Verification items for the finished model (mm, model axes). A direction names the side the tool comes from. Coordinates: 2 decimals unless noted, no trailing zeros. Write each loop counter-clockwise with the first axis right and the second up, starting at its lowest first coordinate (ties: lowest second). Pieces come first, ordered by that corner, then holes. Notation, with made-up numbers: (86.5, 43) - (115.5, 43) arc R33 cw to (115.5, 72) - close; hole circle Ø6 at (74, 3.25). An arc over 180 degrees is marked (long way). Use one line per item in the form item = value. Start each with the question number.
(1) Sectioned sample at B-B (x = 43.05). Record the cut outline in (y, z).
(2) Gauge pin test, flat ends, axial feed: pin 1 Ø1 at (x, y) = (34, 7) entering from +Z; pin 2 Ø0.8 at (y, z) = (8, -11.5) entering from -X; pin 3 Ø3 at (y, z) = (5, 3) entering from +X (3 decimals). Record the tip position at first contact, or that the pin passes through.
(3) Tool access check on faces 1 (the flat face through (25.95, 4, -5)), 2 (the flat face through (36, 5, -12)), 3 (the flat face through (34.05, 10, -6)), 4 (the flat face through (13, 1.5, -5)), 5 (the flat face through (34.05, 4, -6)). Record the directions out of +Z, -Z, +X, -X, +Y, -Y that give a thin tool (end or side, any length) a straight path to the whole face; none if there is none.
(4) Sectioned sample at D-D (x = 0.5). Record the cut outline in (y, z).
(5) Sectioned sample at A-A (y = 3.5). Count the separate pieces of the cut face and the enclosed holes in it, and give its area (3 significant figures).
(6) Sectioned sample at C-C (y = 9.5). Record the cut outline in (x, z) (3 decimals), and give its area (3 significant figures).
(7) Material ranges on line 1 (Z direction, x = 12.5, y = 10.5); line 2 (Z direction, x = 12, y = 0.8); line 3 (X direction, y = 3.6, z = -0.5), recorded low to high. Write a range as [from, to].
(8) Mould release check, pull along Z, two halves, no side actions. Record for faces 6 (the flat face through (36, 5, 1)), 7 (the flat face through (27.18, 0.49, -9.73)), 8 (the flat face through (21.025, 7, -14)): released by +Z, released by -Z, zero draft, split by the parting line, or undercut.
from build123d import *
from build123d.topology import SkipClean

# Parameters (mm, degrees)
ESQUISSE2_W                 = 36.05
ESQUISSE2_H                 = 13
ESQUISSE2_W_2               = 34.05
ESQUISSE2_H_2               = 11
BOSS_EXTRU_1_DEPTH          = 12
ESQUISSE3_W                 = 13
ESQUISSE3_H                 = 1
BOSS_EXTRU_2_DEPTH          = 36.05
ESQUISSE4_R                 = 2.6
ENL_V_MAT_EXTRU_1_DEPTH     = 12
ESQUISSE6_W                 = 3.9
ESQUISSE6_H                 = 1.5
ESQUISSE6_H_2               = 5
ESQUISSE6_H_3               = 7
BOSS_EXTRU_3_DEPTH          = 13
ENL_V_START                 = -6
ENL_V_MAT_EXTRU_2_OUTLINE_R = 0.8
ENL_V_MAT_EXTRU_2_DEPTH     = 6
ESQUISSE8_W                 = 13
ESQUISSE8_H                 = 6.5
ENL_V_MAT_EXTRU_3_DEPTH     = 40.261972696
ESQUISSE9_W                 = 8.1
ESQUISSE9_H                 = 11
BOSS_EXTRU_5_DEPTH          = 1.4
ESQUISSE11_R                = 2.5
ENL_V_MAT_EXTRU_4_DEPTH     = 38.987662471
CONG_2_R                    = 2
ESQUISSE10_W                = 8.1
ESQUISSE10_H                = 11
ENL_V_MAT_EXTRU_5_DEPTH     = 0.8
BOSS_EXTRU_6_DEPTH          = 2.6
ESQUISSE14_R                = 0.5
ENL_V_MAT_EXTRU_7_DEPTH     = 39.645860063
ESQUISSE15_R                = 0.8
ENL_V_MAT_EXTRU_8_DEPTH     = 38.702818197
ESQUISSE16_W                = 3.3
ESQUISSE16_H                = 13
ENL_V_MAT_EXTRU_9_DEPTH     = 1
CHANFREIN1_SIZE             = 0.5
ESQUISSE18_W                = 15
ESQUISSE18_H                = 13
ESQUISSE18_R                = 0.75
BOSS_EXTRU_9_DEPTH          = 5.5
ESQUISSE19_R                = 1.5
BOSS_EXTRU_10_DEPTH         = 12
ENL_V_MAT_EXTRU_10_DEPTH    = 39.061800076
ESQUISSE23_R                = 3.6
ESQUISSE23_R_2              = 2.6
BOSS_EXTRU_11_DEPTH         = 2


# Read off the part's stored shape, not the designer's step: Enlèv. mat.-Extru.2
with BuildPart() as part:
    # Esquisse2 → Boss.-Extru.1 (new body)
    # profile 1 of 3: a face of its own
    with BuildSketch(Plane(origin=(0, 0, 0), x_dir=(1, 0, 0), z_dir=(0, 1, 0))):
        with Locations((17.025, 5.5)):
            Rectangle(ESQUISSE2_W, ESQUISSE2_H)
        with Locations((17.025, 5.5)):
            Rectangle(ESQUISSE2_W_2, ESQUISSE2_H_2, mode=Mode.SUBTRACT)
    # profile 2 of 3: a face of its own
    with BuildSketch(Plane(origin=(0, 0, 0), x_dir=(1, 0, 0), z_dir=(0, 1, 0))):
        Polygon((0, 0), (2.560660172, 0), (0, 2.560660172), align=None)
    # profile 3 of 3: a face of its own
    with BuildSketch(Plane(origin=(0, 0, 0), x_dir=(1, 0, 0), z_dir=(0, 1, 0))):
        Polygon((0, 11), (0, 8.439339828), (2.560660172, 11), align=None)
    extrude(amount=BOSS_EXTRU_1_DEPTH)

    # Esquisse3 → Boss.-Extru.2 (add)
    with BuildSketch(Plane.ZY.offset(1)):
        with Locations((-5.5, 0.5)):
            Rectangle(ESQUISSE3_W, ESQUISSE3_H)
    extrude(amount=-BOSS_EXTRU_2_DEPTH)

    # Esquisse4 → Enlèv. mat.-Extru.1 (cut)
    with BuildSketch(Plane.XZ):
        with Locations(Location((6, -5.5, 0), (0, 0, 270))):
            Circle(ESQUISSE4_R)
        Polygon((34.05, 0), (28.45, 0), (25.95, -2.5), (25.95, -8.5), (28.45, -11), (34.05, -11), align=None)
    extrude(amount=-ENL_V_MAT_EXTRU_1_DEPTH, mode=Mode.SUBTRACT)

    # Esquisse6 → Boss.-Extru.3 (add)
    with BuildSketch(Plane.XY.offset(1)):
        with Locations((12, 0.75)):
            Rectangle(ESQUISSE6_W, ESQUISSE6_H)
        with Locations((18, 2.5)):
            Rectangle(ESQUISSE6_W, ESQUISSE6_H_2)
        with Locations((24, 3.5)):
            Rectangle(ESQUISSE6_W, ESQUISSE6_H_3)
    extrude(amount=-BOSS_EXTRU_3_DEPTH)

    # Enlèv. mat.-Extru.2 outline → Enlèv. mat.-Extru.2 (cut)
    with BuildSketch(Plane(origin=(0, 7, 0), x_dir=(1, 0, 0), z_dir=(0, 1, 0)).offset(ENL_V_START)):
        with BuildLine():
            Line((24, 7.45), (24, 11))
            Line((24, 11), (22.05, 11))
            Line((22.05, 11), (22.05, 5.5))
            ThreePointArc((22.05, 5.5), (22.621141777, 6.878858223), (24, 7.45))
        make_face()
        with BuildLine():
            Line((19.95, 5.5), (19.95, 11))
            Line((19.95, 11), (16.05, 11))
            Line((16.05, 11), (16.05, 5.5))
            ThreePointArc((16.05, 5.5), (18, 7.45), (19.95, 5.5))
        make_face()
        with BuildLine():
            ThreePointArc((24, 3.55), (22.621141777, 4.121141777), (22.05, 5.5))
            Line((22.05, 5.5), (22.05, 0))
            Line((22.05, 0), (24, 0))
            Line((24, 0), (24, 3.55))
        make_face()
        with BuildLine():
            Line((19.95, 0), (19.95, 5.5))
            ThreePointArc((19.95, 5.5), (18, 3.55), (16.05, 5.5))
            Line((16.05, 5.5), (16.05, 0))
            Line((16.05, 0), (19.95, 0))
        make_face()
        with BuildLine():
            Line((13.95, 5.5), (13.95, 11))
            Line((13.95, 11), (10.05, 11))
            Line((10.05, 11), (10.05, 5.5))
            ThreePointArc((10.05, 5.5), (12, 7.45), (13.95, 5.5))
        make_face()
        with BuildLine():
            Line((13.95, 0), (13.95, 5.5))
            ThreePointArc((13.95, 5.5), (12, 3.55), (10.05, 5.5))
            Line((10.05, 5.5), (10.05, 0))
            Line((10.05, 0), (13.95, 0))
        make_face()
        with Locations((24, 5.5)):
            Circle(ENL_V_MAT_EXTRU_2_OUTLINE_R)
        with Locations((18, 5.5)):
            Circle(ENL_V_MAT_EXTRU_2_OUTLINE_R)
        with Locations((12, 5.5)):
            Circle(ENL_V_MAT_EXTRU_2_OUTLINE_R)
    extrude(amount=ENL_V_MAT_EXTRU_2_DEPTH, mode=Mode.SUBTRACT)

    # Esquisse8 → Enlèv. mat.-Extru.3 (cut, through all)
    with BuildSketch(Plane(origin=(0, 0, -12), x_dir=(-1, 0, 0), z_dir=(0, 0, -1))):
        with Locations((-5.5, 8.75)):
            Rectangle(ESQUISSE8_W, ESQUISSE8_H)
    extrude(amount=-ENL_V_MAT_EXTRU_3_DEPTH, mode=Mode.SUBTRACT)

    # Esquisse9 → Boss.-Extru.5 (add)
    with BuildSketch(Plane(origin=(0, 7, 0), x_dir=(1, 0, 0), z_dir=(0, 1, 0))):
        with Locations((30, 5.5)):
            Rectangle(ESQUISSE9_W, ESQUISSE9_H)
        with BuildLine():
            Line((24, 0), (25.95, 0))
            Line((25.95, 0), (25.95, 11))
            Line((25.95, 11), (24, 11))
            Line((24, 11), (24, 7.45))
            Line((24, 7.45), (24, 7.25))
            ThreePointArc((24, 7.25), (25.237436867, 6.737436867), (25.75, 5.5))
            ThreePointArc((25.75, 5.5), (25.237436867, 4.262563133), (24, 3.75))
            Line((24, 3.75), (24, 3.55))
            Line((24, 3.55), (24, 0))
        make_face()
    extrude(amount=BOSS_EXTRU_5_DEPTH)

    # Esquisse11 → Enlèv. mat.-Extru.4 (cut, through all)
    with BuildSketch(Plane(origin=(0, 8.4, 0), x_dir=(1, 0, 0), z_dir=(0, 1, 0))):
        with Locations(Location((30, 5.5, 0), (0, 0, 180))):
            Circle(ESQUISSE11_R)
    extrude(amount=-ENL_V_MAT_EXTRU_4_DEPTH, mode=Mode.SUBTRACT)

    # Congé2
    # the kernel refuses this fillet: 2 mm, written as the material it adds along each edge
    with BuildSketch(Plane(origin=(12, 1, -5.5), x_dir=(-1, 0, 0), z_dir=(0, 0, 1))) as cong_2_piece_1:
        with BuildLine():
            CenterArc((3.272875656, -2), CONG_2_R, 90, 41.409622109)
            Line((1.95, -0.5), (1.95, 0))
            Line((1.95, 0), (3.272875656, 0))
        make_face()
    revolve(axis=Axis((12, 1, -5.5), (0, -1, 0)))
    with BuildSketch(Plane(origin=(18, 1, -5.5), x_dir=(-1, 0, 0), z_dir=(0, 0, 1))) as cong_2_piece_2:
        with BuildLine():
            CenterArc((1.95 + CONG_2_R, -CONG_2_R), CONG_2_R, 90, 90)
            Line((1.95, -CONG_2_R), (1.95, 0))
            Line((1.95, 0), (1.95 + CONG_2_R, 0))
        make_face()
    revolve(axis=Axis((18, 1, -5.5), (0, -1, 0)))
    with BuildSketch(Plane(origin=(24.000000001, 1, -5.500000001), x_dir=(-5.493679582300461e-10, 0, 1.0), z_dir=(1.0, 0, 5.493679582300461e-10))) as cong_2_piece_3:
        with BuildLine():
            CenterArc((1.950000001 + CONG_2_R, -CONG_2_R), CONG_2_R, 90, 90)
            Line((1.950000001, -CONG_2_R), (1.950000001, 0))
            Line((1.950000001, 0), (1.950000001 + CONG_2_R, 0))
        make_face()
    revolve(axis=Axis((24.000000001, 1, -5.500000001), (0, -1, 0)), revolution_arc=89.999999937)
    with BuildSketch(Plane(origin=(24.000000001, 1, -5.499999999), x_dir=(-1.0, 0, -5.49367047277821e-10), z_dir=(-5.49367047277821e-10, 0, 1.0))) as cong_2_piece_4:
        with BuildLine():
            CenterArc((1.950000001 + CONG_2_R, -CONG_2_R), CONG_2_R, 90, 90)
            Line((1.950000001, -CONG_2_R), (1.950000001, 0))
            Line((1.950000001, 0), (1.950000001 + CONG_2_R, 0))
        make_face()
    revolve(axis=Axis((24.000000001, 1, -5.499999999), (0, -1, 0)), revolution_arc=89.999999937)

    # Esquisse10 → Enlèv. mat.-Extru.5 (cut)
    with BuildSketch(Plane.XZ.offset(-7)):
        with Locations((30, -5.5)):
            Rectangle(ESQUISSE10_W, ESQUISSE10_H)
    extrude(amount=-ENL_V_MAT_EXTRU_5_DEPTH, mode=Mode.SUBTRACT)

    # Esquisse13 → Boss.-Extru.6 (add)
    with BuildSketch(Plane(origin=(0, 8.4, 0), x_dir=(1, 0, 0), z_dir=(0, 1, 0))):
        Polygon((34.05, 2.560660172), (31.489339828, 0), (34.05, 0), align=None)
        Polygon((31.489339828, 11), (34.05, 8.439339828), (34.05, 11), align=None)
    extrude(amount=BOSS_EXTRU_6_DEPTH)

    # Esquisse14 → Enlèv. mat.-Extru.7 (cut, through all)
    with BuildSketch(Plane(origin=(0, 11, 0), x_dir=(1, 0, 0), z_dir=(0, 1, 0))):
        with Locations(Location((33.55, 0.5, 0), (0, 0, 270))):
            Circle(ESQUISSE14_R)
        with Locations((33.55, 10.5)):
            Circle(ESQUISSE14_R)
        with Locations(Location((0.5, 0.5, 0), (0, 0, 270))):
            Circle(ESQUISSE14_R)
        with Locations(Location((0.5, 10.5, 0), (0, 0, 270))):
            Circle(ESQUISSE14_R)
    extrude(amount=-ENL_V_MAT_EXTRU_7_DEPTH, mode=Mode.SUBTRACT)

    # Esquisse15 → Enlèv. mat.-Extru.8 (cut, through all)
    with SkipClean():  # the faces are left unmerged after this step: merging them gives an invalid solid
        with BuildSketch(Plane(origin=(0, 7, 0), x_dir=(1, 0, 0), z_dir=(0, 1, 0))):
            with Locations(Location((24, 5.5, 0), (0, 0, 180))):
                Circle(ESQUISSE15_R)
            with Locations(Location((18, 5.5, 0), (0, 0, 180))):
                Circle(ESQUISSE15_R)
            with Locations(Location((12, 5.5, 0), (0, 0, 180))):
                Circle(ESQUISSE15_R)
        extrude(amount=-ENL_V_MAT_EXTRU_8_DEPTH, mode=Mode.SUBTRACT)
    add(part.part.scale(1), mode=Mode.REPLACE)  # the faces are merged on a copy

    # Esquisse16 → Enlèv. mat.-Extru.9 (cut)
    with BuildSketch(Plane(origin=(0, 12, 0), x_dir=(1, 0, 0), z_dir=(0, 1, 0))):
        with Locations((33.4, 5.5)):
            Rectangle(ESQUISSE16_W, ESQUISSE16_H)
    extrude(amount=-ENL_V_MAT_EXTRU_9_DEPTH, mode=Mode.SUBTRACT)

    # Chanfrein1
    chanfrein1_edges = [part.edges().sort_by_distance(p)[0] for p in [
        (24.8, 0, -5.5),
    ]]
    chamfer(chanfrein1_edges, length=CHANFREIN1_SIZE)

    # Esquisse18 → Boss.-Extru.9 (add)
    with BuildSketch(Plane.XZ):
        with Locations((42.55, -5.5)):
            Rectangle(ESQUISSE18_W, ESQUISSE18_H)
        with Locations(Location((43.05, -5.5, 0), (0, 0, 270))):
            Circle(ESQUISSE18_R, mode=Mode.SUBTRACT)
    extrude(amount=-BOSS_EXTRU_9_DEPTH)

    # Esquisse19 → Boss.-Extru.10 (add)
    with BuildSketch(Plane(origin=(0, 12, 0), x_dir=(1, 0, 0), z_dir=(0, 1, 0))):
        with BuildLine():
            Line((28.025, 12), (21.025, 12))
            Line((21.025, 12), (21.025, 18))
            ThreePointArc((21.025, 18), (24.525, 21.5), (28.025, 18))
            Line((28.025, 18), (28.025, 12))
        make_face()
        with Locations(Location((24.525, 18, 0), (0, 0, 270))):
            Circle(ESQUISSE19_R, mode=Mode.SUBTRACT)
    boss_extru_10 = extrude(amount=-BOSS_EXTRU_10_DEPTH)

    # Esquisse21 → Enlèv. mat.-Extru.10 (cut, through all)
    with BuildSketch(Plane(origin=(28.025, 0, 0), x_dir=(0, 0, -1), z_dir=(1, 0, 0))):
        Polygon((12, 0), (16.5, 9), (21.5, 9), (21.5, 0), (16.5, 0), align=None)
    enl_v_mat_extru_10 = extrude(amount=-ENL_V_MAT_EXTRU_10_DEPTH, mode=Mode.SUBTRACT)

    # Esquisse22 → Enlèvement de matière-Révolution1 (revolve, cut)
    with BuildSketch(Plane(origin=(24.525, 0, 0), x_dir=(0, 0, -1), z_dir=(1, 0, 0))):
        Polygon((15.5, 7), (15.5, 9), (16.5, 10), (16.5, 9), (16.5, 7), align=None)
    enl_vement_de_mati_re_r_volution1 = revolve(axis=Axis((24.525, 9, -18), (0, 1, 0)), mode=Mode.SUBTRACT)

    # Symétrie1: Boss.-Extru.10, Enlèv. mat.-Extru.10, Enlèvement de matière-Révolution1 across plane
    add(boss_extru_10.mirror(Plane.XY.offset(-5.5)))
    add(enl_v_mat_extru_10.mirror(Plane.XY.offset(-5.5)), mode=Mode.SUBTRACT)
    add(enl_vement_de_mati_re_r_volution1.mirror(Plane.XY.offset(-5.5)), mode=Mode.SUBTRACT)

    # Esquisse23 → Boss.-Extru.11 (add)
    with BuildSketch(Plane(origin=(0, 1, 0), x_dir=(1, 0, 0), z_dir=(0, 1, 0))):
        with Locations(Location((6, 5.5, 0), (0, 0, 27.702053352))):
            Circle(ESQUISSE23_R)
        with Locations(Location((6, 5.5, 0), (0, 0, 90))):
            Circle(ESQUISSE23_R_2, mode=Mode.SUBTRACT)
    extrude(amount=BOSS_EXTRU_11_DEPTH)


solid = part.part
Answers below:
q1.outline = (0, -12) - (5.5, -12) - (5.5, -6.25) - (0, -6.25) - close; (0, -4.75) - (5.5, -4.75) - (5.5, 1) - (0, 1) - close
q2.pin_1 = 1
q2.pin_2 = 12
q2.pin_3 = 28.025
q3.face_1 = none
q3.face_2 = -Z, +X, +Y, -Y
q3.face_3 = -X, +Y
q3.face_4 = +Y
q3.face_5 = -Y
q4.outline = (0, -12) - (5.5, -12) - (5.5, -11) - (0, -11) - close; (0, -10) - (5.5, -10) - (5.5, -8.94) - (1, -8.94) - (1, -2.06) - (5.5, -2.06) - (5.5, -1) - (0, -1) - close; (0, 0) - (5.5, 0) - (5.5, 1) - (0, 1) - close
q5.separate_pieces = 2
q5.enclosed_holes = 7
q5.area = 352 mm2
q6.outline = (12, -12) - (21.025, -12) - (21.025, -18) arc R3.5 ccw to (28.025, -18) - (28.025, -12) - (35.05, -12) - (35.05, 1) - (28.025, 1) - (28.025, 7) arc R3.5 ccw to (21.025, 7) - (21.025, 1) - (12, 1) - (12, 0) - (31.489, 0) - (34.05, -2.561) - (34.05, -8.439) - (31.489, -11) - (12, -11) - close; hole circle Ø4 at (24.525, -18); hole circle Ø4 at (24.525, 7); hole circle Ø1 at (33.55, -10.5); hole circle Ø1 at (33.55, -0.5)
q6.area = 159 mm2
q7.line_1 = [-12, -11], [0, 1]
q7.line_2 = [-12, -6.3], [-4.7, 1]
q7.line_3 = [-1, 0], [1, 2.06], [24, 25.95], [34.05, 50.05]
q8.face_6 = released by +Z
q8.face_7 = undercut
q8.face_8 = zero draft
